Source: three-view drawing plus pictorial views. Frame: mm from the lowest corner of the part. A direction names the side the tool comes from. Give positions to 0.01 mm unless a question says otherwise; leave off trailing zeros. Loops run counter-clockwise (first coordinate to the right, second up) from the corner with the lowest first, then second, coordinate; pieces in that order, holes last. Notation, with made-up numbers: (76, 75.5) - (121, 75.5) arc R5 ccw to (121, 82.5) - close; hole circle Ø3 at (7.25, -37.75). An arc over 180 degrees is marked (long way). Answer as a JSON object with one key per item and string values.
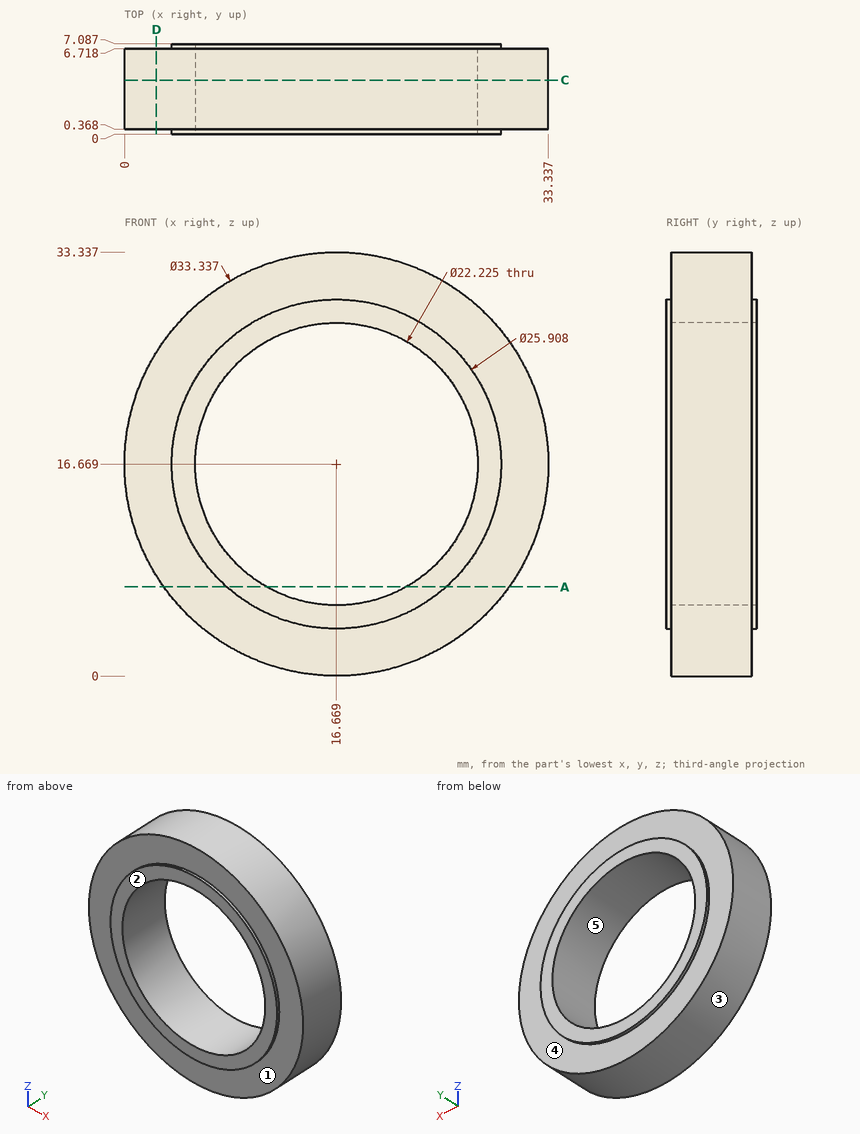
Item 1: Cut plane A-A (z = 7). Return loops of the section in (x, y).
Geometry check:
{"outline": "(3.09, 0.37) - (8.05, 0.37) - (8.05, 0) - (11.19, 0) - (11.19, 7.09) - (8.05, 7.09) - (8.05, 6.72) - (3.09, 6.72) - close; (22.15, 0) - (25.29, 0) - (25.29, 0.37) - (30.25, 0.37) - (30.25, 6.72) - (25.29, 6.72) - (25.29, 7.09) - (22.15, 7.09) - close"}
Item 2: Cut plane D-D (x = 2.5). Return loops of the section in (y, z).
Geometry check:
{"outline": "(0.37, 7.89) - (6.72, 7.89) - (6.72, 25.45) - (0.37, 25.45) - close"}
Item 3: Mould query, pull axis Z, two halves, no side actions, for the marked faces 3, 4 and 5. Classes: released by +Z, released by -Z, zero draft, split by the parting line, or undercut.
Geometry check:
{"face 3": "split by the parting line", "face 4": "zero draft", "face 5": "undercut"}
Item 4: Cut plane C-C (y = 4.25). Return loops of the section in (x, z) (1 decimal).
Geometry check:
{"outline": "circle Ø33.3 at (16.7, 16.7); hole circle Ø22.2 at (16.7, 16.7)"}
Item 5: Contact query for flat-ended pins moving along their axis: P1, Ø4, axis at y = 6, z = 19, coming from the +X side; P2, Ø3, axis at y = 2.5, z = 3.5, coming from the -X side (1 decimal); P3, Ø3, axis at x = 13.5, y = 2.5, coming from the -Z side. Output: stop coordinate, or through.
Geometry check:
{"P1": "stops at x = 33.33", "P2": "stops at x = 4.8", "P3": "stops at z = 0.08"}
Item 6: Material intervals for line 1 (Y direction, x = 13.5, z = 31); line 2 (X direction, y = 1.25, z = 26) (1 decimal); line 3 (X direction, y = 4.5, z = 19) (1 decimal), sorted ascending. Write a range as [from, to].
Geometry check:
{"line 1": "y = [0.37, 6.72]", "line 2": "x = [2.9, 10.6], [22.7, 30.5]", "line 3": "x = [0.2, 5.8], [27.5, 33.2]"}
Item 7: Access query for the marked faces 1 and 2. Directions: +Z, -Z, +X, -X, +Y, -Y. A direction counts if a zero-diameter tool reaches every point of the face in a straight line with its end or side. Return the directions, or none.
Geometry check:
{"face 1": "-Y", "face 2": "+Z, -Z, +X, -X, -Y"}
